For this review, use the dimensioned drawing (mm, ordinates from the lowest corner) and the shaded views. A direction names the side the tool comes from. Give positions to 0.01 mm unless a question says otherwise; leave off trailing zeros. Write each loop counter-clockwise with the first axis right and the second up, starting at its lowest first coordinate (ties: lowest second). Pieces come first, ordered by that corner, then holes.
1) For P1, Ø20.5, axis at x = 25.4, y = 38.1, coming from the -Z side; P2, Ø1, axis at x = 61.5, z = 12, coming from the +Y side; P3, Ø1, axis at x = 33.5, z = 14, coming from the -Y side; P4, Ø7.5, axis at x = 57.15, y = 38.1, coming from the -Z side, all flat-tipped, find the tip position at first contact; note any pin that passes through.
2) Machinability: for the marked faces 5 and 6, which of the approach directions +Z, -Z, +X, -X, +Y, -Y give a long, thin tool a straight path to every point of the face, cutting with its end or side? Answer none if there is none.
3) Wall thickness on line 1 along Y through (x, z) = (25.4, 7.75); line 2 along X through (y, z) = (5.5, 9.5); line 3 along X through (y, z) = (42, 11.5): over which ranges is each line inside the solid? List them lowest first.
4) We need section D-D on x = 57.15. Give the boundary of the cut face in (y, z), and give its area (3 significant figures).
5) We need section C-C on y = 36.5. Give the boundary of the cut face in (x, z), and give its area (3 significant figures).
6) We need section A-A on x = 25.4. Give the boundary of the cut face in (y, z), and give its area (3 significant figures).
7) We need section B-B on z = 9. Give the boundary of the cut face in (x, y), and give its area (3 significant figures).
8) Draft analysis for pull direction Y (two halves, no side actions). For the marked faces 1, 2, 3 and 4, state which applies: pulls with the +Y half, pulls with the -Y half, needs draft (parallel to the pull), parting line crosses it, or undercut.
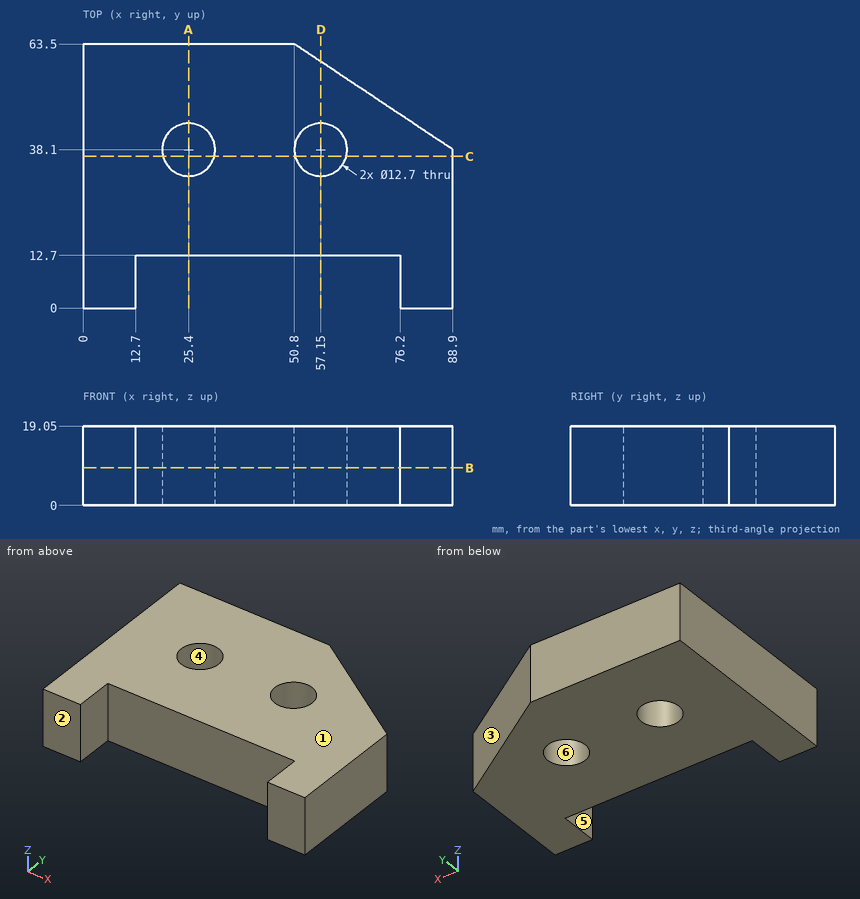
Results list:
1. P1: stops at z = 0
1. P2: stops at y = 56.7
1. P3: stops at y = 12.7
1. P4: passes through
2. face 5: +Z, -Z, -Y
2. face 6: +Z, -Z
3. line 1: y = 12.7 to 31.75, 44.45 to 63.5
3. line 2: x = 0 to 12.7, 76.2 to 88.9
3. line 3: x = 0 to 20.39, 30.41 to 52.14, 62.16 to 83.05
4. outline: (12.7, 0) - (31.75, 0) - (31.75, 19.05) - (12.7, 19.05) - close; (44.45, 0) - (59.27, 0) - (59.27, 19.05) - (44.45, 19.05) - close
4. area: 645 mm2
5. outline: (0, 0) - (19.25, 0) - (19.25, 19.05) - (0, 19.05) - close; (31.55, 0) - (51, 0) - (51, 19.05) - (31.55, 19.05) - close; (63.3, 0) - (88.9, 0) - (88.9, 19.05) - (63.3, 19.05) - close
5. area: 1,230 mm2
6. outline: (12.7, 0) - (31.75, 0) - (31.75, 19.05) - (12.7, 19.05) - close; (44.45, 0) - (63.5, 0) - (63.5, 19.05) - (44.45, 19.05) - close
6. area: 726 mm2
7. outline: (0, 0) - (12.7, 0) - (12.7, 12.7) - (76.2, 12.7) - (76.2, 0) - (88.9, 0) - (88.9, 38.1) - (50.8, 63.5) - (0, 63.5) - close; hole circle Ø12.7 at (25.4, 38.1); hole circle Ø12.7 at (57.15, 38.1)
7. area: 4,100 mm2
8. face 1: needs draft
8. face 2: pulls with the -Y half
8. face 3: pulls with the +Y half
8. face 4: undercut
